```python
from build123d import *

# Parameters (mm, degrees)
BOSS_EXTRUDE1_DEPTH = 12.2
BOSS_EXTRUDE2_DEPTH = 4.3
SKETCH3_R           = 1.5
BOSS_EXTRUDE3_DEPTH = 3.2
SKETCH4_W           = 4.645747774
SKETCH4_H           = 1.682483887
BOSS_EXTRUDE4_DEPTH = 5


with BuildPart() as part:
    # Sketch1 → Boss-Extrude1 (new body)
    with BuildSketch(Plane.XY):
        Polygon((-11.25, 0), (11.25, 0), (11.25, 21), (16.1, 21), (16.1, 23.5), (11.25, 23.5), (11.25, 26.5), (-11.25, 26.5), (-11.25, 23.5), (-16.1, 23.5), (-16.1, 21), (-11.25, 21), align=None)
    extrude(amount=BOSS_EXTRUDE1_DEPTH)

    # Sketch2 → Boss-Extrude2 (add)
    with BuildSketch(Plane(origin=(0, 26.5, 0), x_dir=(1, 0, 0), z_dir=(0, 1, 0))):
        with BuildLine():
            ThreePointArc((-0.298176495, -2.402729564), (-11.25, -6.1), (-0.298176495, -9.797270436))
            ThreePointArc((-0.298176495, -9.797270436), (0.343135361, -9.249221864), (1.153363413, -9.014341819))
            ThreePointArc((1.153363413, -9.014341819), (3.871428575, -6.1), (1.153363413, -3.185658181))
            ThreePointArc((1.153363413, -3.185658181), (0.343135361, -2.950778136), (-0.298176495, -2.402729564))
        make_face()
    extrude(amount=BOSS_EXTRUDE2_DEPTH)

    # Sketch3 → Boss-Extrude3 (add)
    with BuildSketch(Plane(origin=(0, 30.8, 0), x_dir=(1, 0, 0), z_dir=(0, 1, 0))):
        with Locations(Location((-5.15, -6.1, 0), (0, 0, 270))):
            Circle(SKETCH3_R)
    extrude(amount=BOSS_EXTRUDE3_DEPTH)

    # Sketch4 → Boss-Extrude4 (add)
    with BuildSketch(Plane.ZY.offset(11.25)):
        with Locations((6.1, 2.87779749)):
            Rectangle(SKETCH4_W, SKETCH4_H)
    extrude(amount=BOSS_EXTRUDE4_DEPTH)


solid = part.part
```
For this review, take the finished solid that the model builds, in its own axes (mm). A direction names the side the tool comes from. Coordinates: 2 decimals unless noted, no trailing zeros. Write each loop counter-clockwise with the first axis right and the second up, starting at its lowest first coordinate (ties: lowest second). Pieces come first, ordered by that corner, then holes. Notation, with made-up numbers: (77, 74.25) - (105, 74.25) arc R29 cw to (105, 108.25) - close; hole circle Ø10 at (87.5, 79.25). An arc over 180 degrees is marked (long way). Answer in a Markdown table with one row per item. Add a question column.
Q1. For probe 1 along Y at (x, z) = (-2, 5.5); probe 2 along X at (y, z) = (13, 11); probe 3 along Y at (x, z) = (7, 4.75), list the stretches that pass through material, from the lowest coordinate up.
Q2. For P1, Ø1.8, axis at x = -9, z = 3, coming from the +Y side; P2, Ø6, axis at y = 24, z = 10, coming from the -X side; P3, Ø0.5, axis at x = -13.5, y = 2.5, coming from the -Z side, all flat-tipped, find the tip position at first contact; note any pin that passes through.
Q3. We need section C-C, the plane z = 10.5. State the section outline as (x, y) points, and give its area (3 significant figures).
Q4. We need section B-B, the plane y = 17. State the section outline as (x, z) points, and give its area (4 significant figures).
Q5. We need section D-D, the plane x = -2.5. State the section outline as (y, z) points.
Q6. We need section A-A, the plane x = -12. State the section outline as (y, z) points, and give its area (3 significant figures).
Q7. Draft analysis for pull direction Y (two halves, no side actions). For faces 1 (the flat face through (0, 13, 12.2)), 2 (the flat face through (0, 0, 6)), 3 (the flat face through (-14, 3.719, 6)), 4 (the flat face through (-14, 21, 6)), state which applies: +Y half, -Y half, draft (parallel to the pull), parting line (faces both ways), or undercut.
Q8. Tool access review of faces 5 (the cylindrical face through (0.333, 28.62, 9.255)), 6 (the flat face through (-16.1, 22, 6)), 7 (the flat face through (-10, 26.5, 11)), 8 (the cylindrical face through (0.354, 28.62, 2.956)), 9 (the flat face through (-14, 3, 8.423)): name each direction out of +Z, -Z, +X, -X, +Y, -Y from which nothing blocks a thin tool from reaching the whole face with its end or side.
Answer list:
| question | item | result |
|---|---|---|
| 1 | probe 1 | y = 0 to 30.8 |
| 1 | probe 2 | x = -11.25 to 11.25 |
| 1 | probe 3 | y = 0 to 26.5 |
| 2 | P1 | stops at y = 30.8 |
| 2 | P2 | stops at x = -16.1 |
| 2 | P3 | stops at z = 3.78 |
| 3 | outline | (-16.1, 21) - (-11.25, 21) - (-11.25, 0) - (11.25, 0) - (11.25, 21) - (16.1, 21) - (16.1, 23.5) - (11.25, 23.5) - (11.25, 26.5) - (-0.93, 26.5) - (-0.93, 30.8) - (-9.37, 30.8) - (-9.37, 26.5) - (-11.25, 26.5) - (-11.25, 23.5) - (-16.1, 23.5) - close |
| 3 | area | 657 mm2 |
| 4 | outline | (-11.25, 0) - (11.25, 0) - (11.25, 12.2) - (-11.25, 12.2) - close |
| 4 | area | 274.5 mm2 |
| 5 | outline | (0, 0) - (26.5, 0) - (26.5, 0.61) - (30.8, 0.61) - (30.8, 11.59) - (26.5, 11.59) - (26.5, 12.2) - (0, 12.2) - close |
| 6 | outline | (2.04, 3.78) - (3.72, 3.78) - (3.72, 8.42) - (2.04, 8.42) - close; (21, 0) - (23.5, 0) - (23.5, 12.2) - (21, 12.2) - close |
| 6 | area | 38.3 mm2 |
| 7 | face 1 | draft |
| 7 | face 2 | -Y half |
| 7 | face 3 | undercut |
| 7 | face 4 | undercut |
| 8 | face 5 | +Z, +X, +Y |
| 8 | face 6 | +Z, -Z, -X, +Y |
| 8 | face 7 | +Z, -X, +Y |
| 8 | face 8 | -Z, +X, +Y |
| 8 | face 9 | +Z, -X, -Y |
